from build123d import *

# Parameters (mm, degrees)
CYLINDER012_R          = 2
CYLINDER012_DEPTH      = 5.5
CYLINDER013_R          = 2
CYLINDER013_DEPTH      = 5.5
BOX001_W               = 16
BOX001_H               = 10
BOX001_DEPTH           = 31
CYLINDER009_R          = 2.5
CYLINDER009_DEPTH      = 10
CYLINDER008_R          = 6.5
CYLINDER008_DEPTH      = 10
CUT001_PLACEMENT_ANGLE = 90
CYLINDER_R             = 2
CYLINDER_DEPTH         = 2
CYLINDER001_R          = 1
CYLINDER001_DEPTH      = 10
CYLINDER002_R          = 2
CYLINDER002_DEPTH      = 2
CYLINDER003_R          = 1
CYLINDER003_DEPTH      = 10
CYLINDER004_R          = 2
CYLINDER004_DEPTH      = 2
CYLINDER005_R          = 1
CYLINDER005_DEPTH      = 10
CYLINDER006_R          = 2
CYLINDER006_DEPTH      = 2
CYLINDER007_R          = 1
CYLINDER007_DEPTH      = 10
BOX_W                  = 64.27
BOX_H                  = 54.11
BOX_DEPTH              = 3
FILLET_R               = 2
BOX002_W               = 16
BOX002_H               = 10
BOX002_DEPTH           = 31
CYLINDER010_R          = 2.5
CYLINDER010_DEPTH      = 10
CYLINDER011_R          = 6.5
CYLINDER011_DEPTH      = 10
CUT002_PLACEMENT_ANGLE = 90


with BuildPart() as cylinder012:
    # Cylinder012 → Cylinder012 (new body)
    with BuildSketch(Plane(origin=(-15, -17, 0), x_dir=(1, 0, 0), z_dir=(0, 0, 1))):
        Circle(CYLINDER012_R)
    extrude(amount=CYLINDER012_DEPTH)


with BuildPart() as fusion016:
    # Sphere002 → Sphere002 (revolve)
    with BuildSketch(Plane(origin=(-15, -17, 5.5), x_dir=(1, 0, 0), z_dir=(0, -1, 0))):
        with BuildLine():
            ThreePointArc((0, -2), (2, 0), (0, 2))
            Line((0, 2), (0, -2))
        make_face()
    revolve(axis=Axis((-15, -17, 5.5), (0, 0, 1)))

    # Fusion016: union Cylinder012
    add(cylinder012.part)


with BuildPart() as cylinder013:
    # Cylinder013 → Cylinder013 (new body)
    with BuildSketch(Plane(origin=(-15, -17, 0), x_dir=(1, 0, 0), z_dir=(0, 0, 1))):
        Circle(CYLINDER013_R)
    extrude(amount=CYLINDER013_DEPTH)


with BuildPart() as fusion018:
    # Sphere003 → Sphere003 (revolve)
    with BuildSketch(Plane(origin=(-15, -17, 5.5), x_dir=(1, 0, 0), z_dir=(0, -1, 0))):
        with BuildLine():
            ThreePointArc((0, -2), (2, 0), (0, 2))
            Line((0, 2), (0, -2))
        make_face()
    revolve(axis=Axis((-15, -17, 5.5), (0, 0, 1)))

    # Fusion017: union Cylinder013
    add(cylinder013.part)


with BuildPart() as fusion018_1:
    # Fusion017 placement: moved
    add(fusion018.part.moved(Location((30, 0, 0))))

    # Fusion018: union Fusion016
    add(fusion016.part)


with BuildPart() as cube001:
    # Box001 → Box001 (new body)
    with BuildSketch(Plane(origin=(-8, 0, 0), x_dir=(1, 0, 0), z_dir=(0, 0, 1))):
        with Locations((8, 5)):
            Rectangle(BOX001_W, BOX001_H)
    extrude(amount=BOX001_DEPTH)


with BuildPart() as fusion011:
    # Cylinder009 → Cylinder009 (new body)
    with BuildSketch(Plane(origin=(0, -2.5, 0), x_dir=(1, 0, 0), z_dir=(0, 0, 1))):
        Circle(CYLINDER009_R)
    extrude(amount=CYLINDER009_DEPTH)

    # Fusion011: union Cube001
    add(cube001.part)


with BuildPart() as cylinder008:
    # Cylinder008 → Cylinder008 (new body)
    with BuildSketch(Plane.XY):
        Circle(CYLINDER008_R)
    extrude(amount=CYLINDER008_DEPTH)


with BuildPart() as hump:
    # Sphere → Sphere (revolve)
    with BuildSketch(Plane(origin=(0, 0, 10), x_dir=(1, 0, 0), z_dir=(0, -1, 0))):
        with BuildLine():
            ThreePointArc((0, -6.5), (6.5, 0), (0, 6.5))
            Line((0, 6.5), (0, -6.5))
        make_face()
    revolve(axis=Axis((0, 0, 10), (0, 0, 1)))

    # Fusion010: union Cylinder008
    add(cylinder008.part)

    # Cut001: cut Fusion011
    add(fusion011.part, mode=Mode.SUBTRACT)


with BuildPart() as hump_1:
    # Cut001 placement: moved
    add(hump.part.moved(Location((-15, -27.055, 3))).rotate(Axis((-15, -27.055, 3), (-1, 0, 0)), CUT001_PLACEMENT_ANGLE))


with BuildPart() as cylinder:
    # Cylinder → Cylinder (new body)
    with BuildSketch(Plane.XY.offset(2)):
        Circle(CYLINDER_R)
    extrude(amount=CYLINDER_DEPTH)


with BuildPart() as screwhole:
    # Cylinder001 → Cylinder001 (new body)
    with BuildSketch(Plane.XY):
        Circle(CYLINDER001_R)
    extrude(amount=CYLINDER001_DEPTH)

    # Fusion: union Cylinder
    add(cylinder.part)


with BuildPart() as screwhole_1:
    # Fusion placement: moved
    add(screwhole.part.moved(Location((29, 24, 0))))


with BuildPart() as cylinder002:
    # Cylinder002 → Cylinder002 (new body)
    with BuildSketch(Plane.XY.offset(2)):
        Circle(CYLINDER002_R)
    extrude(amount=CYLINDER002_DEPTH)


with BuildPart() as screwhole001:
    # Cylinder003 → Cylinder003 (new body)
    with BuildSketch(Plane.XY):
        Circle(CYLINDER003_R)
    extrude(amount=CYLINDER003_DEPTH)

    # Fusion006: union Cylinder002
    add(cylinder002.part)


with BuildPart() as screwhole001_1:
    # Fusion006 placement: moved
    add(screwhole001.part.moved(Location((-29, 24, 0))))


with BuildPart() as cylinder004:
    # Cylinder004 → Cylinder004 (new body)
    with BuildSketch(Plane.XY.offset(2)):
        Circle(CYLINDER004_R)
    extrude(amount=CYLINDER004_DEPTH)


with BuildPart() as screwhole002:
    # Cylinder005 → Cylinder005 (new body)
    with BuildSketch(Plane.XY):
        Circle(CYLINDER005_R)
    extrude(amount=CYLINDER005_DEPTH)

    # Fusion007: union Cylinder004
    add(cylinder004.part)


with BuildPart() as screwhole002_1:
    # Fusion007 placement: moved
    add(screwhole002.part.moved(Location((29, -24, 0))))


with BuildPart() as cylinder006:
    # Cylinder006 → Cylinder006 (new body)
    with BuildSketch(Plane.XY.offset(2)):
        Circle(CYLINDER006_R)
    extrude(amount=CYLINDER006_DEPTH)


with BuildPart() as screwholes:
    # Cylinder007 → Cylinder007 (new body)
    with BuildSketch(Plane.XY):
        Circle(CYLINDER007_R)
    extrude(amount=CYLINDER007_DEPTH)

    # Fusion008: union Cylinder006
    add(cylinder006.part)


with BuildPart() as screwholes_1:
    # Fusion008 placement: moved
    add(screwholes.part.moved(Location((-29, -24, 0))))

    # Fusion009: union screwHole, screwHole001, screwHole002
    add(screwhole_1.part)
    add(screwhole001_1.part)
    add(screwhole002_1.part)


with BuildPart() as cut:
    # Box → Box (new body)
    with BuildSketch(Plane(origin=(-32.135, -27.055, 0), x_dir=(1, 0, 0), z_dir=(0, 0, 1))):
        with Locations((32.135, 27.055)):
            Rectangle(BOX_W, BOX_H)
    extrude(amount=BOX_DEPTH)

    # Fillet
    fillet_edges = [cut.edges().sort_by_distance(p)[0] for p in [
        (-32.135, -27.055, 1.5),
        (-32.135, 27.055, 1.5),
        (32.135, -27.055, 1.5),
        (32.135, 27.055, 1.5),
    ]]
    fillet(fillet_edges, radius=FILLET_R)

    # Cut: cut ScrewHoles
    add(screwholes_1.part, mode=Mode.SUBTRACT)


with BuildPart() as cube002:
    # Box002 → Box002 (new body)
    with BuildSketch(Plane(origin=(-8, 0, 0), x_dir=(1, 0, 0), z_dir=(0, 0, 1))):
        with Locations((8, 5)):
            Rectangle(BOX002_W, BOX002_H)
    extrude(amount=BOX002_DEPTH)


with BuildPart() as fusion012:
    # Cylinder010 → Cylinder010 (new body)
    with BuildSketch(Plane(origin=(0, -2.5, 0), x_dir=(1, 0, 0), z_dir=(0, 0, 1))):
        Circle(CYLINDER010_R)
    extrude(amount=CYLINDER010_DEPTH)

    # Fusion012: union Cube002
    add(cube002.part)


with BuildPart() as cylinder011:
    # Cylinder011 → Cylinder011 (new body)
    with BuildSketch(Plane.XY):
        Circle(CYLINDER011_R)
    extrude(amount=CYLINDER011_DEPTH)


with BuildPart() as displayback:
    # Sphere001 → Sphere001 (revolve)
    with BuildSketch(Plane(origin=(0, 0, 10), x_dir=(1, 0, 0), z_dir=(0, -1, 0))):
        with BuildLine():
            ThreePointArc((0, -6.5), (6.5, 0), (0, 6.5))
            Line((0, 6.5), (0, -6.5))
        make_face()
    revolve(axis=Axis((0, 0, 10), (0, 0, 1)))

    # Fusion013: union Cylinder011
    add(cylinder011.part)

    # Cut002: cut Fusion012
    add(fusion012.part, mode=Mode.SUBTRACT)


with BuildPart() as displayback_1:
    # Cut002 placement: moved
    add(displayback.part.moved(Location((15, -27.055, 3))).rotate(Axis((15, -27.055, 3), (-1, 0, 0)), CUT002_PLACEMENT_ANGLE))

    # Fusion015: union Hump, Cut
    add(hump_1.part)
    add(cut.part)

    # Cut003: cut Fusion018
    add(fusion018_1.part, mode=Mode.SUBTRACT)


solid = displayback_1.part
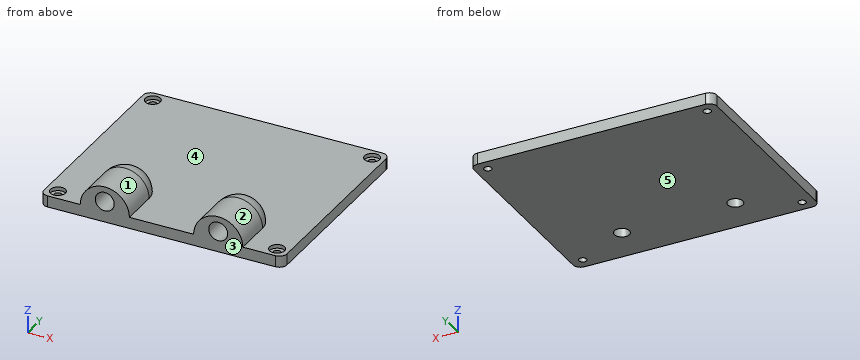
Geometry check sheet. Reference: the model listing, model coordinates, mm. Face numbers are marked on the shaded views. A direction names the side the tool comes from. Give positions to 0.01 mm unless a question says otherwise; leave off trailing zeros. Write each loop counter-clockwise with the first axis right and the second up, starting at its lowest first coordinate (ties: lowest second). Pieces come first, ordered by that corner, then holes.
1) Thickness scan on line 1 (Y direction, x = 29, z = 0.6) (3 decimals); line 2 (Y direction, x = -29, z = 2.7) (3 decimals); line 3 (X direction, y = 24, z = 1.4) (3 decimals). Record the ranges inside material, lowest first.
Values follow:
line 1: y = -27.055 to -25, -23 to 23, 25 to 27.055
line 2: y = -27.055 to -26, -22 to 22, 26 to 27.055
line 3: x = -32.135 to -30, -28 to 28, 30 to 32.135
2) Set-up check for the marked faces 4 and 5: record each of +Z, -Z, +X, -X, +Y, -Y from which the full face is reachable in a straight line by a thin tool's end or side.
Values follow:
face 4: +Z, +Y
face 5: -Z, +X, -X, +Y, -Y
3) Cross-section at B-B (y = 24). Record the boundary of the cut face in (x, z) (3 decimals).
Values follow:
outline: (-32.135, 0) - (-30, 0) - (-30, 2) - (-31, 2) - (-31, 3) - (-32.135, 3) - close; (-28, 0) - (28, 0) - (28, 2) - (27, 2) - (27, 3) - (-27, 3) - (-27, 2) - (-28, 2) - close; (30, 0) - (32.135, 0) - (32.135, 3) - (31, 3) - (31, 2) - (30, 2) - close
4) Release check for a two-part mould opening along X. For the marked faces 1, 2 and 3 record: released by +X, released by -X, zero draft, split by the parting line, or undercut.
Values follow:
face 1: undercut
face 2: undercut
face 3: zero draft
5) Cross-section at C-C (x = 29). Record the boundary of the cut face in (y, z) (3 decimals), plus the area to 3 significant figures.
Values follow:
outline: (-27.055, 0) - (-25, 0) - (-25, 2) - (-26, 2) - (-26, 3) - (-27.055, 3) - close; (-23, 0) - (23, 0) - (23, 2) - (22, 2) - (22, 3) - (-22, 3) - (-22, 2) - (-23, 2) - close; (25, 0) - (27.055, 0) - (27.055, 3) - (26, 3) - (26, 2) - (25, 2) - close
area: 146 mm2
6) Cross-section at A-A (y = -24). Record the boundary of the cut face in (x, z) (3 decimals), plus the area to 3 significant figures.
Values follow:
outline: (-32.135, 0) - (-30, 0) - (-30, 2) - (-31, 2) - (-31, 3) - (-32.135, 3) - close; (-28, 0) - (28, 0) - (28, 2) - (27, 2) - (27, 3) - (21.5, 3) arc R6.5 ccw to (8.5, 3) - (-8.5, 3) arc R6.5 ccw to (-21.5, 3) - (-27, 3) - (-27, 2) - (-28, 2) - close; (30, 0) - (32.135, 0) - (32.135, 3) - (31, 3) - (31, 2) - (30, 2) - close; hole circle Ø5 at (-15, 5.5); hole circle Ø5 at (15, 5.5)
area: 270 mm2
7) Cross-section at D-D (x = 15). Record the boundary of the cut face in (y, z) (3 decimals).
Values follow:
outline: (-27.055, 0) - (-19, 0) - (-19, 3) - (-27.055, 3) - close; (-27.055, 8) - (-17.055, 8) - (-17.055, 7.499) arc R2 cw to (-15, 5.5) - (-15, 0) - (27.055, 0) - (27.055, 3) - (-10.555, 3) arc R6.5 ccw to (-17.055, 9.5) - (-27.055, 9.5) - close
8) Go/stop test with flat-tipped pins: pin 1 Ø2.5 at (x, y) = (-29, 24) entering from +Z; pin 2 Ø3.5 at (x, y) = (-29, 24) entering from -Z; pin 3 Ø12 at (x, y) = (-6.5, 9.5) entering from +Z; pin 4 Ø4.5 at (x, z) = (15, 5.5) entering from -Y (3 decimals). Record where each tip stops, or that it passes through.
Values follow:
pin 1: stops at z = 2
pin 2: stops at z = 0
pin 3: stops at z = 3
pin 4: stops at y = -17.055
